Geometry check sheet. Reference: the model listing, model coordinates, mm. A direction names the side the tool comes from. Round coordinates to 2 decimals unless told otherwise and drop trailing zeros. Order: outer loops, then holes, each group sorted by start corner. A loop starts at its lowest first (then second) coordinate and runs counter-clockwise, first axis right, second up. Notation, with made-up numbers: (-17, -35.5) - (31, -35.5) arc R25 cw to (31, -13.5) - close; hole circle Ø11 at (86.25, 35). An arc over 180 degrees is marked (long way). Write each question's results on one line, items separated by ' | '.
```python
from build123d import *

# Parameters (mm, degrees)
F0_R     = 22.5
F2_R     = 21
F4_R     = 4
F5_R     = 16.25
F6_DEPTH = 21
F7_R     = 4
F8_T     = -1


with BuildPart() as f3:
    # F0 (on Top) → F3 section 0
    with BuildSketch(Plane.XY):
        Circle(F0_R)
    # F2 (on offset) → F3 section 1
    with BuildSketch(Plane.XY.offset(12)):
        Circle(F2_R)
    loft()

    # F4
    f4_edges = [f3.edges().sort_by_distance(p)[0] for p in [
        (-21, 0, 12),
    ]]
    fillet(f4_edges, radius=F4_R)

    # F5 (on face) → F6 (join)
    with BuildSketch(Plane.XY.offset(12)):
        Circle(F5_R)
    extrude(amount=F6_DEPTH)

    # F7
    f7_edges = [f3.edges().sort_by_distance(p)[0] for p in [
        (-16.25, 0, 33),
    ]]
    fillet(f7_edges, radius=F7_R)

    # F8
    f8_openings = [f3.faces().sort_by_distance(p)[0] for p in [
        (0, 0, 0),
    ]]
    offset(amount=F8_T, openings=f8_openings, kind=Kind.INTERSECTION)


solid = f3.part
```
(1) Material ranges on line 1 (Y direction, x = 0, z = 15.75); line 2 (X direction, y = -5, z = 3.5); line 3 (Z direction, x = -6.5, y = -5), recorded low to high.
Answers follow:
line 1: -16.25 to -15.25, 15.25 to 16.25 | line 2: -21.49 to -20.45, 20.45 to 21.49 | line 3: 32 to 33
(2) Section check C-C (z = 6). Record the cut outline in (x, y), then the cut area to 3 significant figures.
Answers follow:
outline: circle Ø43.5 at (0, 0); hole circle Ø41.48 at (0, 0) | area: 135 mm²
(3) Depth check by flat-ended pin: pin 1 Ø10 at (x, z) = (14.5, 21.5) entering from +Y; pin 2 Ø2 at (x, y) = (2, -8) entering from -Z; pin 3 Ø2 at (x, z) = (-3.5, 8.5) entering from +Y. Enter the tip coordinate at first touch or a pass-through.
Answers follow:
pin 1: y = 13.18 | pin 2: z = 32 | pin 3: y = 21.34
(4) Section check A-A (x = 0). Record the cut outline in (y, z), then the cut area to 3 significant figures.
Answers follow:
outline: (-22.5, 0) - (-21.49, 0) - (-20.45, 8.37) arc R3 cw to (-17.47, 11) - (-15.25, 11) - (-15.25, 29) arc R3 cw to (-12.25, 32) - (12.25, 32) arc R3 cw to (15.25, 29) - (15.25, 11) - (17.47, 11) arc R3 cw to (20.45, 8.37) - (21.49, 0) - (22.5, 0) - (21.44, 8.5) arc R4 ccw to (17.47, 12) - (16.25, 12) - (16.25, 29) arc R4 ccw to (12.25, 33) - (-12.25, 33) arc R4 ccw to (-16.25, 29) - (-16.25, 12) - (-17.47, 12) arc R4 ccw to (-21.44, 8.5) - close | area: 101 mm²
(5) Section check B-B (z = 27). Record the cut outline in (x, y).
Answers follow:
outline: circle Ø32.5 at (0, 0); hole circle Ø30.5 at (0, 0)
(6) Access from +Z, -Z, +X, -X, +Y, -Y to the whole of each face (thin tool, end or side, straight path). Record for faces 5 (the face through (-12.1, -9.28, 19.87)), 6 (the face through (0, 0, 33)), 7 (the face through (12, -12, 12)).
Answers follow:
face 5: -Z | face 6: +Z, +X, -X, +Y, -Y | face 7: +Z
(7) Draft check along X on faces 1 (the face through (-2.683, 20.437, 7.035)), 2 (the face through (1, 16, 11)), 3 (the face through (-2.813, 21.424, 7.14)), 4 (the face through (22, -2, 0)). Enter one of: released by +X, released by -X, zero draft, split by the parting line, or undercut.
Answers follow:
face 1: undercut | face 2: undercut | face 3: split by the parting line | face 4: zero draft
